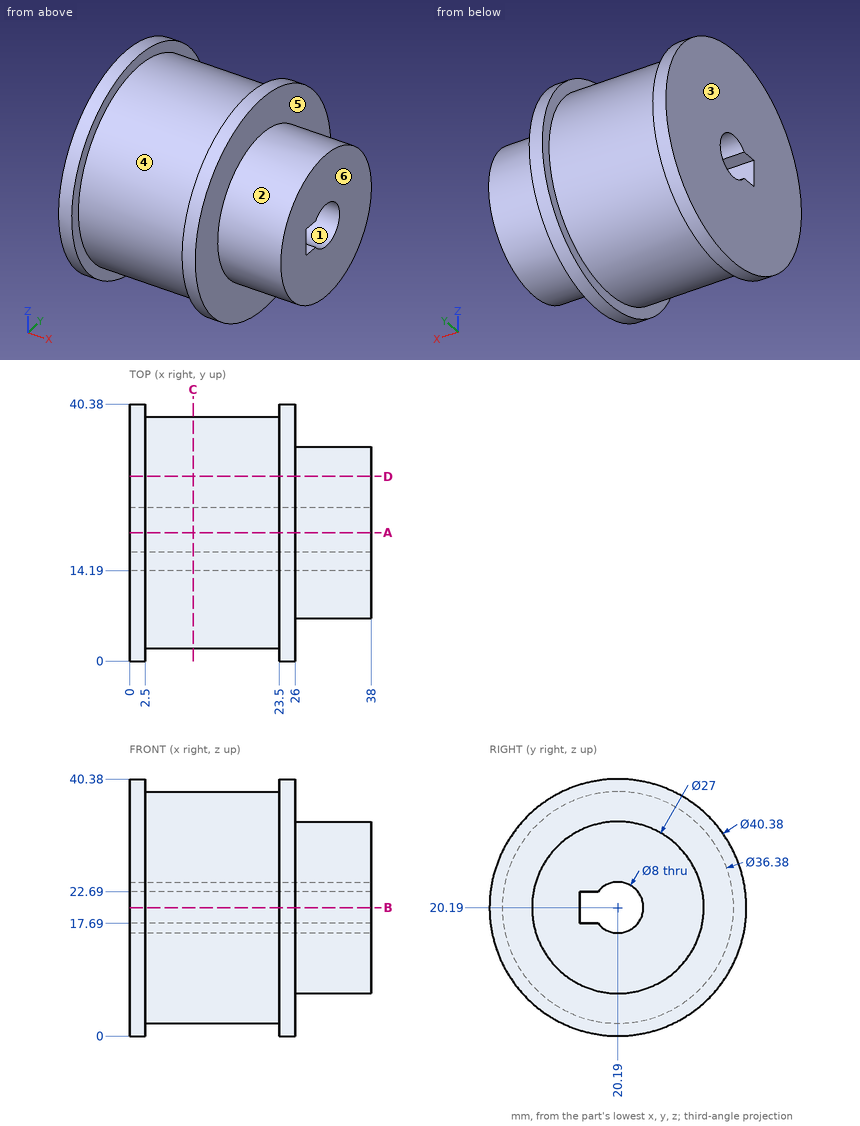
Study the drawing (mm; zero at the part's minimum x, y, z) and answer. A direction names the side the tool comes from. Coordinates: 2 decimals unless noted, no trailing zeros. Write each loop counter-clockwise with the first axis right and the second up, starting at its lowest first coordinate (ties: lowest second). Pieces come first, ordered by that corner, then holes.
Q1. Which of the six approach directions +Z, -Z, +X, -X, +Y, -Y give full straight-line access (tool end or side, diameter ignored) to the marked faces 4, 5 and 6?
Returned:
face 4: none
face 5: +X
face 6: +Z, -Z, +X, +Y, -Y
Q2. Find the intervals of material crossed by line 1 along Y through (x, z) = (12, 20); line 2 along Z through (x, y) = (29, 20.19); line 3 along X through (y, z) = (17.5, 2), in increasing order.
Returned:
line 1: y = 2 to 14.19, 24.19 to 38.38
line 2: z = 6.69 to 16.19, 24.19 to 33.69
line 3: x = 0 to 2.5, 23.5 to 26
Q3. Given P1, Ø10, axis at x = 28.5, y = 24, coming from the -Z side; P2, Ø5, axis at x = 32.5, y = 10.5, coming from the -Z side; P3, Ø1.4, axis at x = 24.5, y = 16, coming from the +Z side; P4, Ø5, axis at x = 30.5, z = 32.5, coming from the -Y side, each flat-ended and moving along its own axis, determine where each tip first touches the part or whether it passes through.
Returned:
P1: stops at z = 0
P2: stops at z = 8.76
P3: stops at z = 40.08
P4: stops at y = 10.92
Q4. Section A-A, the plane y = 20.19 is taken. Write down the section's boundary in (x, z).
Returned:
outline: (0, 0) - (2.5, 0) - (2.5, 2) - (23.5, 2) - (23.5, 0) - (26, 0) - (26, 6.69) - (38, 6.69) - (38, 16.19) - (0, 16.19) - close; (0, 24.19) - (38, 24.19) - (38, 33.69) - (26, 33.69) - (26, 40.38) - (23.5, 40.38) - (23.5, 38.38) - (2.5, 38.38) - (2.5, 40.38) - (0, 40.38) - close
Q5. The mould has two halves that part along Y. Classify the marked faces 1, 2 and 3: released by +Y, released by -Y, zero draft, split by the parting line, or undercut.
Returned:
face 1: undercut
face 2: split by the parting line
face 3: zero draft
Q6. Section C-C, the plane x = 10 is taken. Write down the section's boundary in (y, z).
Returned:
outline: circle Ø36.38 at (20.19, 20.19); hole (14.19, 17.69) - (17.07, 17.69) arc R4 ccw (long way) to (17.07, 22.69) - (14.19, 22.69) - close
Q7. Section B-B, the plane z = 20.19 is taken. Write down the section's boundary in (x, y), then the cut area to 3 significant figures.
Returned:
outline: (0, 0) - (2.5, 0) - (2.5, 2) - (23.5, 2) - (23.5, 0) - (26, 0) - (26, 6.69) - (38, 6.69) - (38, 14.19) - (0, 14.19) - close; (0, 24.19) - (38, 24.19) - (38, 33.69) - (26, 33.69) - (26, 40.38) - (23.5, 40.38) - (23.5, 38.38) - (2.5, 38.38) - (2.5, 40.38) - (0, 40.38) - close
area: 910 mm2
Q8. Section D-D, the plane y = 29 is taken. Write down the section's boundary in (x, z), then the cut area to 3 significant figures.
Returned:
outline: (0, 2.02) - (2.5, 2.02) - (2.5, 4.28) - (23.5, 4.28) - (23.5, 2.02) - (26, 2.02) - (26, 9.96) - (38, 9.96) - (38, 30.42) - (26, 30.42) - (26, 38.36) - (23.5, 38.36) - (23.5, 36.1) - (2.5, 36.1) - (2.5, 38.36) - (0, 38.36) - close
area: 1,100 mm2
